Design review of the part shown in the three views and the two pictorial views. Dimensions are in mm from the part's minimum x, y and z. A direction names the side the tool comes from. Give positions to 0.01 mm unless a question says otherwise; leave off trailing zeros. Order: outer loops, then holes, each group sorted by start corner. A loop starts at its lowest first (then second) coordinate and runs counter-clockwise, first axis right, second up.
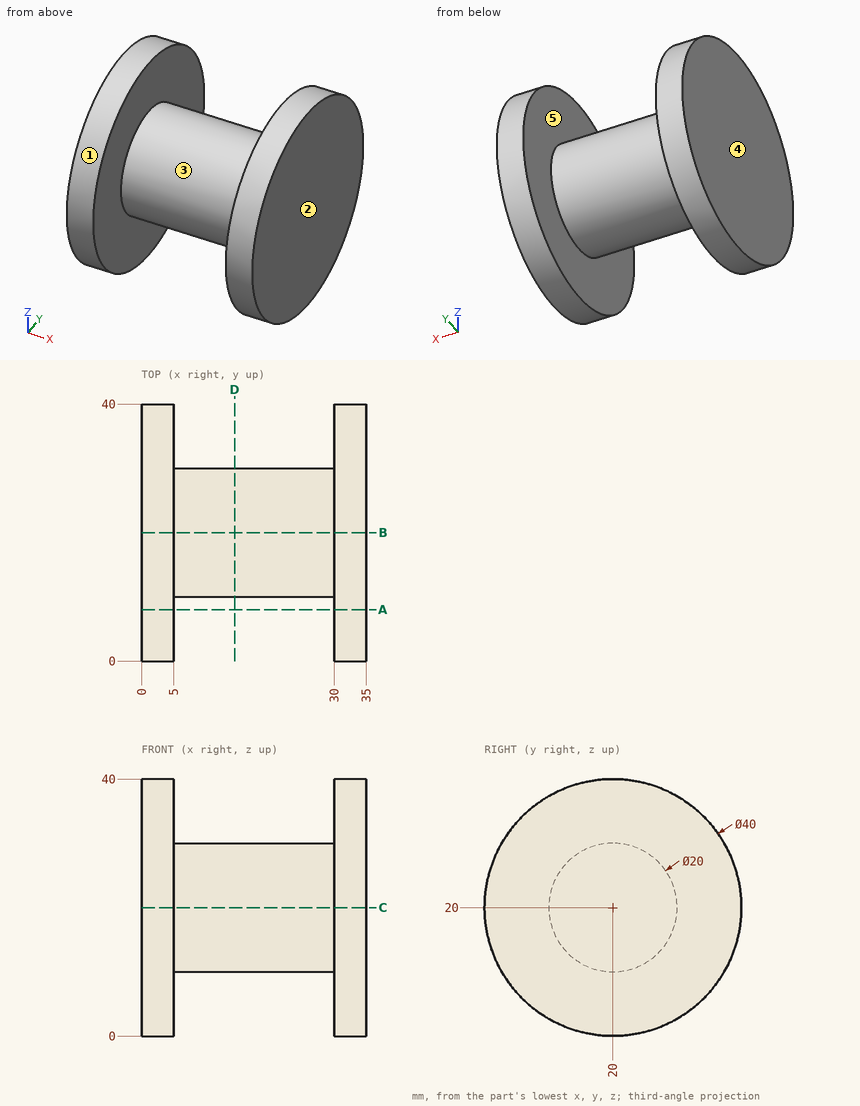
1) We need section B-B on y = 20. Give the boundary of the cut face in (x, z), then the cut area to 3 significant figures.
Answer sheet:
outline: (0, 0) - (5, 0) - (5, 10) - (30, 10) - (30, 0) - (35, 0) - (35, 40) - (30, 40) - (30, 30) - (5, 30) - (5, 40) - (0, 40) - close
area: 900 mm2
2) Draft analysis for pull direction X (two halves, no side actions). For the marked faces 1, 2 and 3, state which applies: +X half, -X half, draft (parallel to the pull), parting line (faces both ways), or undercut.
Answer sheet:
face 1: draft
face 2: +X half
face 3: undercut
3) Tool access review of the marked faces 4 and 5: name each direction out of +Z, -Z, +X, -X, +Y, -Y from which nothing blocks a thin tool from reaching the whole face with its end or side.
Answer sheet:
face 4: +Z, -Z, -X, +Y, -Y
face 5: none
4) Clearance check with flat-ended pins moving along their axes: pin 1 (8 mm diameter, centred on x = 20, y = 22.5, fed in from +Z); pin 2 (6 mm diameter, centred on y = 28, z = 19.5, fed in from -X); pin 3 (10 mm diameter, centred on x = 22.5, z = 16.5, fed in from -Y); pin 4 (2 mm diameter, centred on x = 31, z = 35, fed in from -Y). State where each tip first meets the part, or that it passes through.
Answer sheet:
pin 1: stops at z = 30
pin 2: stops at x = 0
pin 3: stops at y = 10
pin 4: stops at y = 5.72
5) To check wall thickness, follow line 1 (X direction, y = 33.5, z = 7.5); line 2 (Z direction, x = 7, y = 20); line 3 (Z direction, x = 18, y = 29). State the ranges of each line that lie inside material, in increasing order.
Answer sheet:
line 1: x = 0 to 5, 30 to 35
line 2: z = 10 to 30
line 3: z = 15.64 to 24.36
6) We need section D-D on x = 14.5. Give the boundary of the cut face in (y, z), then the cut area to 3 significant figures.
Answer sheet:
outline: circle Ø20 at (20, 20)
area: 314 mm2
7) We need section A-A on y = 8. Give the boundary of the cut face in (x, z).
Answer sheet:
outline: (0, 4) - (5, 4) - (5, 36) - (0, 36) - close; (30, 4) - (35, 4) - (35, 36) - (30, 36) - close
